CAD build for the part. Positions are in the model's coordinates, mm. A direction names the side the tool comes from. Round coordinates to 2 decimals unless told otherwise and drop trailing zeros. Write each loop counter-clockwise with the first axis right and the second up, starting at its lowest first coordinate (ties: lowest second). Pieces come first, ordered by that corner, then holes. Notation, with made-up numbers: (-2, -39) - (38, -39) arc R21 cw to (38, -9) - close; hole circle Ø2 at (85, -25). An arc over 180 degrees is marked (long way). Answer in a Markdown table with one row per item.
Autodesk Inventor part; units mm, degrees
ref_plane "YZ Plane" through (0, 0, 0) normal (1, 0, 0) x (0, 1, 0)
ref_plane "XZ Plane" through (0, 0, 0) normal (0, 1, 0) x (-1, 0, 0)
ref_plane "XY Plane" through (0, 0, 0) normal (0, 0, 1) x (1, 0, 0)
sketch "Sketch1" plane through (0, 0, 0) normal (0, 0, 1) x (1, 0, 0)
  circle A0 centre (0, 0) radius 8
  line L0 (1, 7.9373) -> (40.375, 2.9765)
  line L1 (1, -7.9373) -> (40.375, -2.9765)
  line L2 (0, 0) -> (40, 0) construction
  circle A1 centre (40, 0) radius 3
  circle A2 centre (-6.0777, -34.4683) radius 2.5
  line L3 (-3.7145, -35.2839) -> (7.5623, -2.61)
  line L4 (-8.5773, -34.4264) -> (-7.9989, 0.1339)
  line L5 (0, 0) -> (-6.0777, -34.4683) construction
  circle A3 centre (-25.9808, 15) radius 3.5
  line L6 (-24.7052, 18.2593) -> (2.9155, 7.4498)
  line L7 (-4.994, -6.2498) -> (-28.1656, 12.2657)
  line L8 (-25.9808, 15) -> (0, 0) construction
  point P0 (-3.8416, -33.3502)
  dimension "d0" = 16
  dimension "d1" = 6
  dimension "d2" = 40
  dimension "d3" = 5
  dimension "d4" = 35
  dimension "d5" = 100
  dimension "d32" = 18.082
  dimension "d36" = 30
  dimension "d37" = 7
  dimension "d38" = 150
extrude "Extrusion1" add sketch "Sketch1" along normal blind 3
fillet "Fillet1" radius 5 3 edges at (5.9384, -7.3151, 1.5) (1.9881, 7.8128, 1.5) (-8.0647, -3.7962, 1.5)
sketch "Sketch2" plane through (0, 0, 3) normal (0, 0, 1) x (1, 0, 0)
  point P0 (0, 0)
  point P1 (0, 0)
hole "Hole1" at (0, 0, 3) direction (0, 0, -1) diameter 6.2 end through all
sketch "Sketch3" plane through (0, 0, 3) normal (0, 0, 1) x (1, 0, 0)
  line L0 (-8.1058, -6.2524) -> (-8.5773, -34.4264)
  line L1 (-3.7145, -35.2839) -> (4.9235, -10.2558)
  point P0 (0, 0)
  point P1 (-3.473, -19.6962)
  point P2 (-7.4498, 2.9155)
  point P3 (-8.5773, -34.4264)
  point P4 (-9.2276, -1.6271)
  dimension "d33" = 20
  dimension "d34" = 4.8571
  dimension "d35" = 4.8571
hole "Hole2" [suppressed]
sketch "Sketch4" plane through (0, 0, 3) normal (0, 0, 1) x (1, 0, 0)
  arc A0 (-8.5773, -34.4264) -> (-3.7145, -35.2839) centre (-6.0777, -34.4683) ccw
  arc A1 (-24.7052, 18.2593) -> (-28.1656, 12.2657) centre (-25.9808, 15) ccw
  point P0 (0, 0)
hole "Hole3" at (-25.9808, 15, 3) direction (0, 0, -1) diameter 3 end through all
properties part number "Pancake_Switch Lever 2" material "Nylon 6/6"
Q1. Flat gauge pin, fed straight in: pin 1 (1.5 mm diameter, centred on x = 29.5, z = 2.5, fed in from +Y). Where does the tip first touch, or does it go through?
Computed:
| item | result |
|---|---|
| pin 1 | stops at y = 4.44 |
Q2. Saw through at C-C on x = 0. List the corners of the cut face in (y, z).
Computed:
| item | result |
|---|---|
| outline | (-24.52, 0) - (-3.1, 0) - (-3.1, 3) - (-24.52, 3) - close; (3.1, 0) - (8.59, 0) - (8.59, 3) - (3.1, 3) - close |
Q3. 3-axis set-ups, long thin cutter, end or side, ignore diameter. For faces 1 (the flat face through (4, -1, 3)), 2 (the cylindrical face through (-8.568, -4.068, 1.521)): which of +Z, -Z, +X, -X, +Y, -Y reach the whole face in a straight line?
Computed:
| item | result |
|---|---|
| face 1 | +Z, +X, -X, +Y, -Y |
| face 2 | +Z, -Z, -X |
Q4. Pull direction Y, two halves, no side cores. Call faces 3 (the cylindrical face through (-29.046, 16.689, 1.479)), 4 (the cylindrical face through (2.75, -1.43, 1.48)), 5 (the flat face through (21.23, 5.39, 1.48)): released by +Y, released by -Y, zero draft, split by the parting line, or undercut.
Computed:
| item | result |
|---|---|
| face 3 | split by the parting line |
| face 4 | undercut |
| face 5 | released by +Y |
Q5. Saw through at D-D on x = -15. List the corners of the cut face in (y, z).
Computed:
| item | result |
|---|---|
| outline | (1.75, 0) - (14.46, 0) - (14.46, 3) - (1.75, 3) - close |
Q6. Saw through at A-A on y = 0. List the corners of the cut face in (x, z).
Computed:
| item | result |
|---|---|
| outline | (-12.82, 0) - (-3.1, 0) - (-3.1, 3) - (-12.82, 3) - close; (3.1, 0) - (43, 0) - (43, 3) - (3.1, 3) - close |
Q7. Saw through at B-B on z = 1.2. List the corners of the cut face in (x, y) (1 decimal).
Computed:
| item | result |
|---|---|
| outline | (-28.2, 12.3) - (-10, -2.3) arc R5 cw to (-8.1, -6.3) - (-8.6, -34.4) arc R2.5 ccw to (-3.7, -35.3) - (4.9, -10.3) arc R5 cw to (9, -6.9) - (40.4, -3) arc R3 ccw to (40.4, 3) - (2.6, 7.7) arc R5 cw to (1.4, 8) - (-24.7, 18.3) arc R3.5 ccw to start; hole circle Ø3 at (-26, 15); hole circle Ø6.2 at (0, 0) |
Q8. Drill centre lines: line 1 (X direction, y = 0, z = 1); line 2 (X direction, y = 1.5, z = 2.5); line 3 (X direction, y = -7.5, z = 2.45). Where is each one in solid material? Low to high.
Computed:
| item | result |
|---|---|
| line 1 | x = -12.82 to -3.1, 3.1 to 43 |
| line 2 | x = -14.69 to -2.71, 2.71 to 42.6 |
| line 3 | x = -8.13 to 7.25 |
